Verification items for this drawing (mm, ordinates from the low corner). A direction names the side the tool comes from. Coordinates: 2 decimals unless noted, no trailing zeros. Order: outer loops, then holes, each group sorted by start corner. A loop starts at its lowest first (then second) coordinate and runs counter-clockwise, first axis right, second up. Notation, with made-up numbers: M 14.25,39.25 L 33.25,39.25 A33 ccw 33.25,72.25 Z; hole C 5,20.25 d6. An arc over 180 degrees is marked long. Answer as a JSON object with one key per item and string values. Group by question number.
(1) Access from +Z, -Z, +X, -X, +Y, -Y to the whole of each face (thin tool, end or side, straight path). Record for the marked faces 3, 4 and 5.
(2) Cross-section at C-C (z = 5). Enter the section's corners in (x, y), plus the area to 3 significant figures.
(3) Cross-section at A-A (y = 0.5). Enter the section's corners in (x, z).
(4) Cross-section at D-D (x = 18.5). Enter the section's corners in (y, z).
(5) Material ranges on line 1 (Z direction, x = 1, y = 2.9); line 2 (Y direction, x = 13.75, z = 4.5); line 3 (X direction, y = 0.5, z = 4.5), recorded low to high.
(6) Gauge pin test, flat ends, axial feed: pin 1 Ø0.5 at (y, z) = (1, 5) entering from -X; pin 2 Ø0.9 at (y, z) = (1.5, 3.5) entering from +X. Record the tip position at first contact, or that the pin passes through.
(7) Mould release check, pull along X, two halves, no side actions. Record for the marked faces 1 and 2: released by +X, released by -X, zero draft, split by the parting line, or undercut.
(8) Cross-section at B-B (y = 2.5). Enter the section's corners in (x, z), plus the area to 3 significant figures.
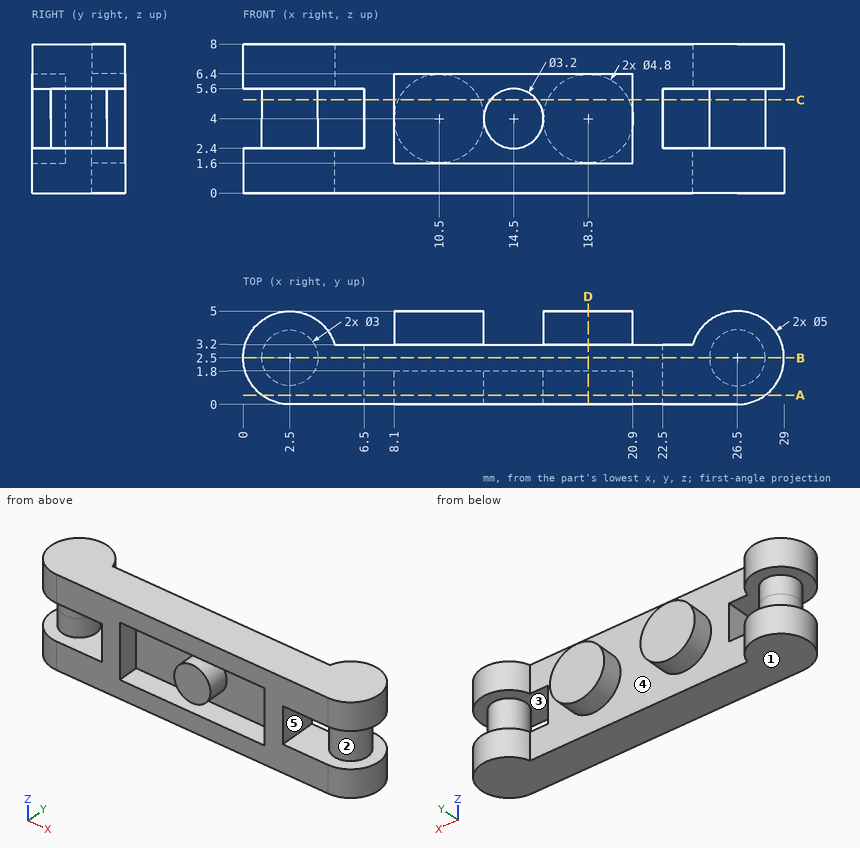
Taken from the geometry:
{
 "1": {"face 3": "none", "face 4": "+Y", "face 5": "+Y, -Y"},
 "2": {"outline": "C 2.5,2.5 d3; M 6.5,0 L 8.1,0 L 8.1,1.8 L 13.25,1.8 L 13.25,0 L 15.75,0 L 15.75,1.8 L 20.9,1.8 L 20.9,0 L 22.5,0 L 22.5,3.2 L 20.68,3.2 L 20.68,5 L 16.32,5 L 16.32,3.2 L 12.68,3.2 L 12.68,5 L 8.32,5 L 8.32,3.2 L 6.5,3.2 Z; C 26.5,2.5 d3", "area": "62.5 mm²"},
 "3": {"outline": "M 1,0 L 28,0 L 28,2.4 L 22.5,2.4 L 22.5,5.6 L 28,5.6 L 28,8 L 1,8 L 1,5.6 L 6.5,5.6 L 6.5,2.4 L 1,2.4 Z; C 14.5,4 d3.2; hole M 8.1,1.6 L 20.9,1.6 L 20.9,6.4 L 8.1,6.4 Z"},
 "4": {"outline": "M 0,0 L 3.2,0 L 3.2,1.6 L 5,1.6 L 5,6.4 L 3.2,6.4 L 3.2,8 L 0,8 L 0,6.4 L 1.8,6.4 L 1.8,1.6 L 0,1.6 Z"},
 "5": {"line 1": "z = 0 to 2.4, 5.6 to 8", "line 2": "y = 0 to 3.2", "line 3": "x = 6.5 to 8.1, 12.98 to 16.02, 20.9 to 22.5"},
 "6": {"pin 1": "stops at x = 1.67", "pin 2": "stops at x = 27.9"},
 "7": {"face 1": "zero draft", "face 2": "undercut"},
 "8": {"outline": "M 0,0 L 29,0 L 29,2.4 L 28,2.4 L 28,5.6 L 29,5.6 L 29,8 L 0,8 L 0,5.6 L 1,5.6 L 1,2.4 L 0,2.4 Z; hole M 4,2.4 L 6.5,2.4 L 6.5,5.6 L 4,5.6 Z; hole M 22.5,2.4 L 25,2.4 L 25,5.6 L 22.5,5.6 Z", "area": "210 mm²"}
}
